Read the model definition and answer for the solid it produces. Units are mm, in the model's axes. A direction names the side the tool comes from. Round coordinates to 2 decimals unless told otherwise and drop trailing zeros. Loops run counter-clockwise (first coordinate to the right, second up) from the corner with the lowest first, then second, coordinate; pieces in that order, holes last. Notation, with made-up numbers: M -26.75,53.5 L 17.25,53.5 A23 cw 17.25,64.5 Z; hole C 23,17.25 d6. An arc over 180 degrees is marked long. Write each question's results on one line, items separated by ' | '.
from build123d import *

# Parameters (mm, degrees)
BASE_FLANGE1_DEPTH           = 50
CUT_EXTRUDE1_REACH           = 92.111
SKETCH23_R                   = 11.04
SKETCH23_R_2                 = 1.75
CUT_EXTRUDE2_REACH           = 90.414
CHAMFER1_SIZE                = 5.5
TALADRO_DE_MARGEN_PARA_M31_D = 3.4
MATRIZC1_COUNT               = 4


# Sheet-metal steps are written as plain solids
with BuildPart() as part:
    # Sketch2 → Base-Flange1 (new body)
    with BuildSketch(Plane(origin=(0, 0, 0), x_dir=(-1, 0, 0), z_dir=(0, 0, -1))):
        with BuildLine():
            Line((0, 52), (0, 3.7366))
            ThreePointArc((0, 3.7366), (-1.094424801, 1.094424801), (-3.7366, 0))
            Line((-3.7366, 0), (-54, 0))
            Line((-54, 0), (-54, 3))
            Line((-54, 3), (-3.7366, 3))
            ThreePointArc((-3.7366, 3), (-3.215745145, 3.215745145), (-3, 3.7366))
            Line((-3, 3.7366), (-3, 52))
            Line((-3, 52), (0, 52))
        make_face()
    extrude(amount=BASE_FLANGE1_DEPTH)

    # Sketch23 → Cut-Extrude1 (cut, up to next)
    with BuildSketch(Plane.ZY, mode=Mode.PRIVATE) as cut_extrude1_sk1:
        with Locations(Location((-25, 30, 0), (0, 0, 270))):
            Circle(SKETCH23_R)
    cut_extrude1_tool1 = extrude(cut_extrude1_sk1.sketch, amount=-CUT_EXTRUDE1_REACH, mode=Mode.PRIVATE) & part.part
    # Sketch23 → Cut-Extrude1 (cut, up to next)
    with BuildSketch(Plane.ZY, mode=Mode.PRIVATE) as cut_extrude1_sk2:
        with Locations(Location((-9.5, 45.5, 0), (0, 0, 270))):
            Circle(SKETCH23_R_2)
    cut_extrude1_tool2 = extrude(cut_extrude1_sk2.sketch, amount=-CUT_EXTRUDE1_REACH, mode=Mode.PRIVATE) & part.part
    # Sketch23 → Cut-Extrude1 (cut, up to next)
    with BuildSketch(Plane.ZY, mode=Mode.PRIVATE) as cut_extrude1_sk3:
        with Locations(Location((-9.5, 14.5, 0), (0, 0, 270))):
            Circle(SKETCH23_R_2)
    cut_extrude1_tool3 = extrude(cut_extrude1_sk3.sketch, amount=-CUT_EXTRUDE1_REACH, mode=Mode.PRIVATE) & part.part
    # Sketch23 → Cut-Extrude1 (cut, up to next)
    with BuildSketch(Plane.ZY, mode=Mode.PRIVATE) as cut_extrude1_sk4:
        with Locations(Location((-40.5, 14.5, 0), (0, 0, 270))):
            Circle(SKETCH23_R_2)
    cut_extrude1_tool4 = extrude(cut_extrude1_sk4.sketch, amount=-CUT_EXTRUDE1_REACH, mode=Mode.PRIVATE) & part.part
    # Sketch23 → Cut-Extrude1 (cut, up to next)
    with BuildSketch(Plane.ZY, mode=Mode.PRIVATE) as cut_extrude1_sk5:
        with Locations(Location((-40.5, 45.5, 0), (0, 0, 270))):
            Circle(SKETCH23_R_2)
    cut_extrude1_tool5 = extrude(cut_extrude1_sk5.sketch, amount=-CUT_EXTRUDE1_REACH, mode=Mode.PRIVATE) & part.part
    add(cut_extrude1_tool1.solids().sort_by_distance((0, 30, -25))[0], mode=Mode.SUBTRACT)
    add(cut_extrude1_tool2.solids().sort_by_distance((0, 45.5, -9.5))[0], mode=Mode.SUBTRACT)
    add(cut_extrude1_tool3.solids().sort_by_distance((0, 14.5, -9.5))[0], mode=Mode.SUBTRACT)
    add(cut_extrude1_tool4.solids().sort_by_distance((0, 14.5, -40.5))[0], mode=Mode.SUBTRACT)
    add(cut_extrude1_tool5.solids().sort_by_distance((0, 45.5, -40.5))[0], mode=Mode.SUBTRACT)

    # Sketch24 → Cut-Extrude2 (cut, up to next)
    with BuildSketch(Plane(origin=(0, 3, 0), x_dir=(1, 0, 0), z_dir=(0, 1, 0)), mode=Mode.PRIVATE) as cut_extrude2_sk1:
        with BuildLine():
            Line((42, 7.85), (12, 7.85))
            ThreePointArc((12, 7.85), (9.85, 10), (12, 12.15))
            Line((12, 12.15), (42, 12.15))
            ThreePointArc((42, 12.15), (44.15, 10), (42, 7.85))
        make_face()
    cut_extrude2_tool1 = extrude(cut_extrude2_sk1.sketch, amount=-CUT_EXTRUDE2_REACH, mode=Mode.PRIVATE) & part.part
    # Sketch24 → Cut-Extrude2 (cut, up to next)
    with BuildSketch(Plane(origin=(0, 3, 0), x_dir=(1, 0, 0), z_dir=(0, 1, 0)), mode=Mode.PRIVATE) as cut_extrude2_sk2:
        with BuildLine():
            Line((12, 42.15), (42, 42.15))
            ThreePointArc((42, 42.15), (44.15, 40), (42, 37.85))
            Line((42, 37.85), (12, 37.85))
            ThreePointArc((12, 37.85), (9.85, 40), (12, 42.15))
        make_face()
    cut_extrude2_tool2 = extrude(cut_extrude2_sk2.sketch, amount=-CUT_EXTRUDE2_REACH, mode=Mode.PRIVATE) & part.part
    add(cut_extrude2_tool1.solids().sort_by_distance((27, 3, -10))[0], mode=Mode.SUBTRACT)
    add(cut_extrude2_tool2.solids().sort_by_distance((27, 3, -40))[0], mode=Mode.SUBTRACT)

    # Chamfer1
    chamfer1_edges = [part.edges().sort_by_distance(p)[0] for p in [
        (1.5, 52, -50),
        (54, 1.5, -50),
        (1.5, 52, 0),
        (54, 1.5, 0),
    ]]
    chamfer(chamfer1_edges, length=CHAMFER1_SIZE)

    # Taladro de margen para M31 (through all)
    with Locations(Plane.ZY):
        with Locations((-15.100505063, 39.899494937)):
            taladro_de_margen_para_m31 = Hole(TALADRO_DE_MARGEN_PARA_M31_D / 2)

    # MatrizC1: Taladro de margen para M31 ×4 about axis
    matrizc1_axis = Axis((0, 30, -25), (1, 0, 0))
    for i in range(1, MATRIZC1_COUNT):
        add(taladro_de_margen_para_m31.rotate(matrizc1_axis, i * 360 / MATRIZC1_COUNT), mode=Mode.SUBTRACT)


solid = part.part
Item 1: The part is cut by section A-A (x = 28.5). Determine the outline of the cut face in (y, z).
Outcome:
outline: M 0,-50 L 3,-50 L 3,-42.15 L 0,-42.15 Z; M 0,-37.85 L 3,-37.85 L 3,-12.15 L 0,-12.15 Z; M 0,-7.85 L 3,-7.85 L 3,0 L 0,0 Z
Item 2: Flat-ended cylindrical pins translate along their axes: pin 1 (5.5 mm diameter, centred on y = 39.9, z = -34.9, fed in from -X); pin 2 (25 mm diameter, centred on x = 33.5, z = -13, fed in from +Y). Find the tip coordinate at first contact, or state that the pin passes through.
Outcome:
pin 1: stops at x = 0 | pin 2: stops at y = 3
Item 3: Straight lines are drawn through the part: line 1 (Z direction, x = 1.6, y = 14.5); line 2 (Y direction, x = 2, z = -40); line 3 (X direction, y = 7, z = -34.5). For each, find the intervals that lie inside material, in ascending order.
Outcome:
line 1: z = -50 to -42.25, -38.75 to -11.25, -7.75 to 0 | line 2: y = 0.43 to 12.82, 16.18 to 43.82, 47.18 to 52 | line 3: x = 0 to 3
Item 4: The part is cut by section D-D (z = -6.5). Determine the outline of the cut face in (x, y), plus the area to 3 significant figures.
Outcome:
outline: M 0,3.74 A3.74 ccw 3.74,0 L 54,0 L 54,3 L 3.74,3 A0.74 cw 3,3.74 L 3,52 L 0,52 Z | area: 306 mm2
Item 5: For faces 5 (the face through (27, 2, -7.85)), 6 (the face through (1.07, 1.12, -24.65)), 7 (the face through (29, 3, -25)), determine the directions among +Z, -Z, +X, -X, +Y, -Y from which every point of the face is accessible in a straight line to the end or side of a thin tool.
Outcome:
face 5: +Y, -Y | face 6: +Z, -Z, -X, -Y | face 7: +Z, -Z, +X, +Y
Item 6: The mould has two halves that part along Z. Classify faces 1 (the face through (51.3, 1.5, -2.8)), 2 (the face through (2, 52, -25)), 3 (the face through (1.5, 49.2, -47.3)), 4 (the face through (44.15, 1.52, -10.05)): pulls with the +Z half, pulls with the -Z half, needs draft (parallel to the pull), parting line crosses it, or undercut.
Outcome:
face 1: pulls with the +Z half | face 2: needs draft | face 3: pulls with the -Z half | face 4: undercut
Item 7: The part is cut by section B-B (y = 45.5). Determine the outline of the cut face in (x, z).
Outcome:
outline: M 0,-50 L 3,-50 L 3,-42.25 L 0,-42.25 Z; M 0,-38.75 L 3,-38.75 L 3,-11.25 L 0,-11.25 Z; M 0,-7.75 L 3,-7.75 L 3,0 L 0,0 Z
Item 8: The part is cut by section C-C (z = -25). Determine the outline of the cut face in (x, y).
Outcome:
outline: M 0,3.74 A3.74 ccw 3.74,0 L 54,0 L 54,3 L 3.74,3 A0.74 cw 3,3.74 L 3,18.96 L 0,18.96 Z; M 0,41.04 L 3,41.04 L 3,52 L 0,52 Z
